Source: CAD feature listing. Evaluate the final solid. Frame: model axes, mm. A direction names the side the tool comes from. Give positions to 0.01 mm unless a question says otherwise; leave off trailing zeros. Order: outer loops, then holes, each group sorted by start corner. A loop starts at its lowest first (then second) coordinate and runs counter-clockwise, first axis right, second up.
1) First-contact query: P1, Ø2, axis at y = 137, z = -133.5, coming from the +X side; P2, Ø12, axis at y = 127, z = -92.5, coming from the -X side; P3, Ø15.5, axis at x = -21.5, z = -179, coming from the +Y side. Flat tips, straight axial feed; report the tip coordinate or a pass-through.
2) Access query for faces 4 (the face through (-4, 40.6, -184.8)), 5 (the face through (0, 79, -94)), 6 (the face through (-32, 41, -185)), 7 (the face through (145.77, 78.88, -16.28)), 8 (the face through (-32, 41, -189)). Directions: +Z, -Z, +X, -X, +Y, -Y. A direction counts if a zero-diameter tool reaches every point of the face in a straight line with its end or side. Return the directions, or none.
3) Material intervals for line 1 (Z direction, x = 175, y = 59.5); line 2 (X direction, y = 142, z = -37); line 3 (X direction, y = 53.5, z = -132.5), sorted ascending.
4) Section D-D, the plane z = -86.5. Return loops of the section in (x, y).
5) Section A-A, the plane z = -24.5. Return loops of the section in (x, y), plus the area to 3 significant figures.
6) Section C-C, the plane x = 67. Return loops of the section in (y, z), plus the area to 3 significant figures.
7) Section B-B, the plane y = 74.5. Return loops of the section in (x, z).
8) Draft query along Z for faces 1 (the face through (-7.01, 40.56, -182.15)), 2 (the face through (67, 160, 0.3)), 3 (the face through (91, 79, 0)). Return one class per face: released by +Z, released by -Z, zero draft, split by the parting line, or undercut.
```python
from build123d import *

# Parameters (mm, degrees)
BASE_FLANGE3_DEPTH = 160
EDGE_FLANGE4_DEPTH = 80
HEM1_DEPTH         = 160


# Read off the part's stored shape, not the designer's step: Hem1
# Sheet-metal steps are written as plain solids
with BuildPart() as part:
    # Sketch1 → Base-Flange3 (new body)
    with BuildSketch(Plane(origin=(0, 0, 0), x_dir=(1, 0, 0), z_dir=(0, 1, 0))):
        with BuildLine():
            Line((0, 175), (0, 10))
            ThreePointArc((0, 10), (2.928932188, 2.928932188), (10, 0))
            Line((10, 0), (175, 0))
            Line((175, 0), (175, -4))
            Line((175, -4), (10, -4))
            ThreePointArc((10, -4), (0.100505063, 0.100505063), (-4, 10))
            Line((-4, 10), (-4, 175))
            Line((-4, 175), (0, 175))
        make_face()
    extrude(amount=BASE_FLANGE3_DEPTH)

    # Edge-Flange4 section (across the edge) → Edge-Flange4 (add)
    with BuildSketch(Plane(origin=(-4, 80, -185), x_dir=(0, 0, 1), z_dir=(0, -1, 0))):
        with BuildLine():
            Line((-4, 10), (-4, 46))
            Line((-4, 46), (0, 46))
            Line((0, 46), (0, 10))
            ThreePointArc((0, 10), (2.928932188, 2.928932188), (10, 0))
            Line((10, 0), (10, -4))
            ThreePointArc((10, -4), (0.100505063, 0.100505063), (-4, 10))
        make_face()
    extrude(amount=EDGE_FLANGE4_DEPTH)

    # Hem1 outline → Hem1 (add)
    with BuildSketch(Plane(origin=(0, 0, 0), x_dir=(1, 0, 0), z_dir=(0, 1, 0))):
        with BuildLine():
            Line((129.174241339, 2.724359327), (132.238419112, 0.153208889))
            Line((132.238419112, 0.153208889), (159.679111138, 32.855752194))
            ThreePointArc((159.679111138, 32.855752194), (193.126155741, 28.452365235), (175, 0))
            Line((175, 0), (175, -4))
            ThreePointArc((175, -4), (196.751386889, 30.142838282), (156.614933365, 35.426902632))
            Line((156.614933365, 35.426902632), (129.174241339, 2.724359327))
        make_face()
    extrude(amount=HEM1_DEPTH)


solid = part.part
```
From the geometry:
1. P1: stops at x = 0
1. P2: stops at x = -4
1. P3: stops at y = 80
2. face 4: -Z, +X, +Y, -Y
2. face 5: -Z, +Y, -Y
2. face 6: +Z, -X, +Y, -Y
2. face 7: +Y, -Y
2. face 8: -Z, +X, -X, +Y, -Y
3. line 1: z = -44 to -40, 0 to 4
3. line 2: x = -4 to 0, 158.06 to 164.46, 185.54 to 191.94
3. line 3: x = -4 to 0
4. outline: (-4, 0) - (0, 0) - (0, 160) - (-4, 160) - close
5. outline: (-4, 0) - (0, 0) - (0, 160) - (-4, 160) - close; (147.45, 0) - (152.67, 0) - (152.67, 160) - (147.45, 160) - close; (194.49, 0) - (198.57, 0) - (198.57, 160) - (194.49, 160) - close
5. area: 2,130 mm2
6. outline: (0, 0) - (160, 0) - (160, 4) - (0, 4) - close
6. area: 640 mm2
7. outline: (-50, -189) - (-14, -189) arc R14 ccw to (0, -175) - (0, -10) arc R10 cw to (10, 0) - (175, 0) arc R20 cw (long way) to (159.68, -32.86) - (132.24, -0.15) - (129.17, -2.72) - (156.61, -35.43) arc R24 ccw (long way) to (175, 4) - (10, 4) arc R14 ccw to (-4, -10) - (-4, -175) arc R10 cw to (-14, -185) - (-50, -185) - close
8. face 1: released by +Z
8. face 2: zero draft
8. face 3: undercut
